Read the model definition and answer for the solid it produces. Units are mm, in the model's axes. A direction names the side the tool comes from. Coordinates: 2 decimals unless noted, no trailing zeros. Loops run counter-clockwise (first coordinate to the right, second up) from the corner with the lowest first, then second, coordinate; pieces in that order, holes last. Notation, with made-up numbers: (56, 61.25) -> (62, 61.25) arc R8 ccw to (62, 71.25) -> close; hole circle Ø4 at (66, 26). An arc over 180 degrees is marked (long way). Answer as a JSON object with one key per item and string values. Group by question number.
1) Which of the six approach directions +Z, -Z, +X, -X, +Y, -Y give full straight-line access (tool end or side, diameter ignored) to faces 4 (the face through (6, 8, 5)), 5 (the face through (6, -3, 5)), 6 (the face through (14, 0, 1)), 7 (the face through (6, -8, 5))?
2) Section B-B, the plane x = 9.75 is taken. Give the vertices of the cut face in (y, z), plus the area to 3 significant figures.
3) Section D-D, the plane y = 4 is taken. Give the vertices of the cut face in (x, z).
4) Determine the mould class of faces 1 (the face through (9.5, 1.35, 3.8)), 2 (the face through (14, -6, 1)), 3 (the face through (0, -9, 5)) for opening direction Y: released by +Y, released by -Y, zero draft, split by the parting line, or undercut.
5) Flat-ended cylindrical pins translate along their axes: P1, Ø5, axis at x = 12, z = 6.5, coming from the -Y side; P2, Ø1.5, axis at y = 4.5, z = 5.5, coming from the +X side; P3, Ø0.8, axis at y = -8.5, z = 4, coming from the +X side; P4, Ø5, axis at x = 12.5, z = 4, coming from the +Y side. Find the tip coordinate at first contact, or state that the pin passes through.
6) Section C-C, the plane x = -3.25 is taken. Give the vertices of the cut face in (y, z), plus the area to 3 significant figures.
7) Consider probe 1 along Y at (x, z) = (13.5, 7); probe 2 along Z at (x, y) = (11, -5.95); probe 3 along X at (y, z) = (-8, 6.25). Determine where each line is inside the solid, lowest interval first. Write a range as [from, to].
from build123d import *

# Parameters (mm, degrees)
F0_W     = 10
F0_H     = 2.9
F1_DEPTH = 10
F2_R     = 3.05
F3_DEPTH = 8
F4_R     = 1.55
F5_DEPTH = 25
F6_R     = 0.5
F7_R     = 4.99999


# Not quite as in the source:
# - a fillet or chamfer is up to 0.001 mm smaller than in the source, because OpenCascade refuses the exact size


with BuildPart() as f1:
    # F0 (on Top) → F1 (new body)
    with BuildSketch(Plane.XY):
        Polygon((6, 9), (-6, 9), (-6, -9), (6, -9), (6, -7.55), (6, -4.65), (6, -1.55), (6, 1.35), (6, 4.45), (6, 7.35), align=None)
        with Locations((11, 5.9)):
            Rectangle(F0_W, F0_H)
        with Locations((11, -0.1)):
            Rectangle(F0_W, F0_H)
        with Locations((11, -6.1)):
            Rectangle(F0_W, F0_H)
    extrude(amount=F1_DEPTH)

    # F2 (on face) → F3 (cut)
    with BuildSketch(Plane(origin=(-6, 0, 0), x_dir=(0, -1, 0), z_dir=(-1, 0, 0))):
        with Locations((0, 5)):
            Circle(F2_R)
    extrude(amount=-F3_DEPTH, mode=Mode.SUBTRACT)

    # F4 (on face) → F5 (cut)
    with BuildSketch(Plane.XZ.offset(7.55)):
        with Locations((11, 5)):
            Circle(F4_R)
    extrude(amount=-F5_DEPTH, mode=Mode.SUBTRACT)

    # F6
    f6_edges = [f1.edges().sort_by_distance(p)[0] for p in [
        (-6, 0, 10),
        (0, -9, 10),
        (0, 9, 10),
        (-6, -9, 5),
        (-6, 0, 0),
        (-6, 9, 5),
        (0, 9, 0),
        (0, -9, 0),
        (6, -9, 5),
        (6, -8.275, 0),
        (6, -3.1, 0),
        (6, 2.9, 0),
        (6, 8.175, 0),
        (6, 9, 5),
        (6, 8.175, 10),
        (6, 2.9, 10),
        (6, -3.1, 10),
        (6, -8.275, 10),
    ]]
    fillet(f6_edges, radius=F6_R)

    # F7 (radius 5 in the source; OpenCascade refuses exactly that, so slightly less here)
    f7_edges = [f1.edges().sort_by_distance(p)[0] for p in [
        (16, 5.9, 0),
        (16, 5.9, 10),
        (16, -0.1, 10),
        (16, -0.1, 0),
        (16, -6.1, 0),
        (16, -6.1, 10),
    ]]
    fillet(f7_edges, radius=F7_R)


solid = f1.part
Determined:
{
 "1": {"face 4": "+Z, -Z, +X, +Y", "face 5": "+Z, -Z, +X", "face 6": "-Z, +X, +Y, -Y", "face 7": "+Z, -Z, +X, -Y"},
 "2": {"outline": "(-7.55, 0) -> (-4.65, 0) -> (-4.65, 4.08) -> (-7.55, 4.08) -> close; (-7.55, 5.92) -> (-4.65, 5.92) -> (-4.65, 10) -> (-7.55, 10) -> close; (-1.55, 0) -> (1.35, 0) -> (1.35, 4.08) -> (-1.55, 4.08) -> close; (-1.55, 5.92) -> (1.35, 5.92) -> (1.35, 10) -> (-1.55, 10) -> close; (4.45, 0) -> (7.35, 0) -> (7.35, 4.08) -> (4.45, 4.08) -> close; (4.45, 5.92) -> (7.35, 5.92) -> (7.35, 10) -> (4.45, 10) -> close", "area": "71.1 mm²"},
 "3": {"outline": "(-6, 0.5) arc R0.5 ccw to (-5.5, 0) -> (5.5, 0) arc R0.5 ccw to (6, 0.5) -> (6, 9.5) arc R0.5 ccw to (5.5, 10) -> (-5.5, 10) arc R0.5 ccw to (-6, 9.5) -> close"},
 "4": {"face 1": "undercut", "face 2": "zero draft", "face 3": "released by -Y"},
 "5": {"P1": "y = -7.55", "P2": "x = 16", "P3": "x = 6", "P4": "y = 7.35"},
 "6": {"outline": "(-9, 0.5) arc R0.5 ccw to (-8.5, 0) -> (8.5, 0) arc R0.5 ccw to (9, 0.5) -> (9, 9.5) arc R0.5 ccw to (8.5, 10) -> (-8.5, 10) arc R0.5 ccw to (-9, 9.5) -> close; hole circle Ø6.1 at (0, 5)", "area": "151 mm²"},
 "7": {"probe 1": "[-7.55, -4.65], [-1.55, 1.35], [4.45, 7.35]", "probe 2": "[0, 3.45], [6.55, 10]", "probe 3": "[-6, 6]"}
}
